Input: part model. Units: mm. Frame: model coordinates. Give positions to 0.01 mm unless a question says otherwise; leave off trailing zeros. Order: outer loops, then holes, each group sorted by start corner. A loop starts at its lowest first (then second) coordinate and runs counter-clockwise, first axis right, second up. Notation, with made-up numbers: M 4.5,-36 L 55.5,-36 A10 ccw 55.5,-25 Z; hole C 17.5,48 d1. An arc over 180 degrees is marked long. Use a Markdown table: item, result.
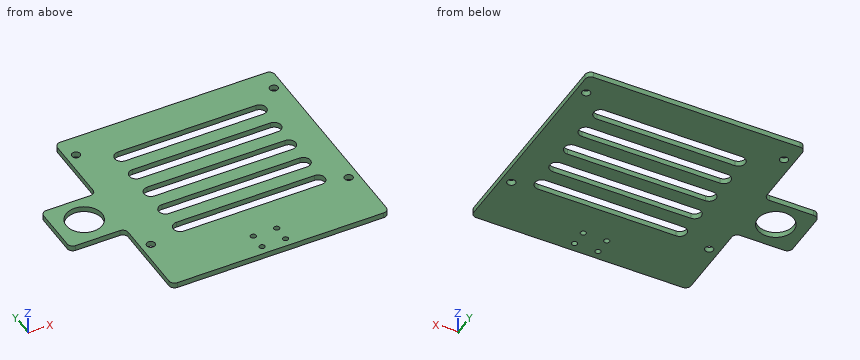
Autodesk Fusion 360 part; units mm, degrees
sketch "Sketch1" plane through (0, 0, 0) normal (0, 0, 1) x (1, 0, 0)
  line L0 (-78.5381, -2.5381) -> (-78.5381, 7.765)
  line L1 (-76.5381, 58.0111) -> (-1.7619, 58.0111)
  line L2 (0.2381, 56.0111) -> (0.2381, -2.5381)
  circle A0 centre (-3.3, -1) radius 1.5
  circle A1 centre (-3.3, 50) radius 1.5
  circle A2 centre (-75, 50) radius 1.5
  circle A3 centre (-75, -1) radius 1.5
  line L3 (-62.5, 45) -> (-12.5, 45)
  line L4 (-12.5, 40) -> (-62.5, 40)
  line L5 (-62.5, 35) -> (-12.5, 35)
  line L6 (-12.5, 30) -> (-62.5, 30)
  line L7 (-62.5, 25) -> (-12.5, 25)
  line L8 (-12.5, 20) -> (-62.5, 20)
  line L9 (-62.5, 15) -> (-12.5, 15)
  line L10 (-12.5, 10) -> (-62.5, 10)
  line L11 (-62.5, 5) -> (-12.5, 5)
  line L12 (-12.5, 0) -> (-62.5, 0)
  arc A4 (-62.5, 45) -> (-65, 42.5) centre (-62.5, 42.5) ccw
  arc A5 (-65, 42.5) -> (-62.5, 40) centre (-62.5, 42.5) ccw
  arc A6 (-10, 42.5) -> (-12.5, 45) centre (-12.5, 42.5) ccw
  arc A7 (-12.5, 40) -> (-10, 42.5) centre (-12.5, 42.5) ccw
  arc A8 (-62.5, 35) -> (-65, 32.5) centre (-62.5, 32.5) ccw
  arc A9 (-65, 32.5) -> (-62.5, 30) centre (-62.5, 32.5) ccw
  arc A10 (-10, 32.5) -> (-12.5, 35) centre (-12.5, 32.5) ccw
  arc A11 (-12.5, 30) -> (-10, 32.5) centre (-12.5, 32.5) ccw
  arc A12 (-10, 22.5) -> (-12.5, 25) centre (-12.5, 22.5) ccw
  arc A13 (-12.5, 20) -> (-10, 22.5) centre (-12.5, 22.5) ccw
  arc A14 (-62.5, 25) -> (-65, 22.5) centre (-62.5, 22.5) ccw
  arc A15 (-65, 22.5) -> (-62.5, 20) centre (-62.5, 22.5) ccw
  arc A16 (-62.5, 15) -> (-65, 12.5) centre (-62.5, 12.5) ccw
  arc A17 (-65, 12.5) -> (-62.5, 10) centre (-62.5, 12.5) ccw
  arc A18 (-10, 12.5) -> (-12.5, 15) centre (-12.5, 12.5) ccw
  arc A19 (-12.5, 10) -> (-10, 12.5) centre (-12.5, 12.5) ccw
  arc A20 (-10, 2.5) -> (-12.5, 5) centre (-12.5, 2.5) ccw
  arc A21 (-12.5, 0) -> (-10, 2.5) centre (-12.5, 2.5) ccw
  arc A22 (-62.5, 5) -> (-65, 2.5) centre (-62.5, 2.5) ccw
  arc A23 (-65, 2.5) -> (-62.5, 0) centre (-62.5, 2.5) ccw
  line L13 (-80.5381, 29.765) -> (-96.5381, 29.765)
  line L14 (-98.5381, 27.765) -> (-98.5381, 11.765)
  line L15 (-96.5381, 9.765) -> (-80.5381, 9.765)
  circle A24 centre (-88, 20) radius 6.5
  arc A25 (-76.5381, 58.0111) -> (-78.5381, 56.0111) centre (-76.5381, 56.0111) ccw
  arc A26 (0.2381, 56.0111) -> (-1.7619, 58.0111) centre (-1.7619, 56.0111) ccw
  arc A27 (-78.5381, 7.765) -> (-80.5381, 9.765) centre (-80.5381, 7.765) ccw
  arc A28 (-96.5381, 29.765) -> (-98.5381, 27.765) centre (-96.5381, 27.765) ccw
  arc A29 (-98.5381, 11.765) -> (-96.5381, 9.765) centre (-96.5381, 11.765) ccw
  line L16 (-78.5381, 56.0111) -> (-78.5381, 31.765)
  arc A30 (-80.5381, 29.765) -> (-78.5381, 31.765) centre (-80.5381, 31.765) ccw
  line L17 (0.2381, -2.5381) -> (0.2381, -19.9889)
  line L18 (-1.7619, -21.9889) -> (-76.5381, -21.9889)
  line L19 (-78.5381, -19.9889) -> (-78.5381, -2.5381)
  arc A31 (-78.5381, -19.9889) -> (-76.5381, -21.9889) centre (-76.5381, -19.9889) ccw
  arc A32 (-1.7619, -21.9889) -> (0.2381, -19.9889) centre (-1.7619, -19.9889) ccw
  circle A33 centre (-44.1028, -12.7273) radius 1
  circle A34 centre (-35.6028, -12.7273) radius 1
  circle A35 centre (-35.6028, -18.7273) radius 1
  circle A36 centre (-44.1028, -18.7273) radius 1
  point P0 (-98.5381, 29.765)
  dimension "d1" = 71.7
  dimension "d2" = 51
  dimension "d4" = 3
  dimension "d5" = 3
  dimension "d6" = 3
  dimension "d7" = 3
  dimension "d8" = 2.5
  dimension "d9" = 2.5
  dimension "d18" = 13
  dimension "d21" = 2
  dimension "d22" = 2
  dimension "d25" = 2
  dimension "d28" = 80
  dimension "d37" = 8.5
  dimension "d38" = 6
  dimension "d39" = 2
  dimension "d40" = 2
  dimension "d41" = 2
  dimension "d42" = 2
extrude "Extrude4" add sketch "Sketch1" along normal blind 2
1) Cut plane D-D on z = 1.65. State how many separate pieces and enclosed holes the cut face has, and give its area (3 significant figures).
Response values:
| item | result |
|---|---|
| separate pieces | 1 |
| enclosed holes | 14 |
| area | 5,180 mm² |
2) Cut plane C-C on y = 22.5. Return loops of the section in (x, z), and give its area (3 significant figures).
Response values:
| item | result |
|---|---|
| outline | M -98.54,0 L -94,0 L -94,2 L -98.54,2 Z; M -82,0 L -65,0 L -65,2 L -82,2 Z; M -10,0 L 0.24,0 L 0.24,2 L -10,2 Z |
| area | 63.6 mm² |
3) Cut plane A-A on y = 50. Return loops of the section in (x, z), and give its area (3 significant figures).
Response values:
| item | result |
|---|---|
| outline | M -78.54,0 L -76.5,0 L -76.5,2 L -78.54,2 Z; M -73.5,0 L -4.8,0 L -4.8,2 L -73.5,2 Z; M -1.8,0 L 0.24,0 L 0.24,2 L -1.8,2 Z |
| area | 146 mm² |
4) Material intervals for line 1 (Y direction, x = -56, z = 1.15); line 2 (Y direction, x = -88.5, z = 0.35) (3 decimals); line 3 (X direction, y = 21, z = 1), sorted ascending. Write a range as from..to.
Response values:
| item | result |
|---|---|
| line 1 | y = -21.99..0, 5..10, 15..20, 25..30, 35..40, 45..58.01 |
| line 2 | y = 9.765..13.519, 26.481..29.765 |
| line 3 | x = -98.54..-94.42, -81.58..-64.5, -10.5..0.24 |
5) Cut plane B-B on y = 2.5. Return loops of the section in (x, z).
Response values:
| item | result |
|---|---|
| outline | M -78.54,0 L -65,0 L -65,2 L -78.54,2 Z; M -10,0 L 0.24,0 L 0.24,2 L -10,2 Z |
6) First-contact query: pin 1 Ø2.5 at (x, y) = (-75, -1) entering from -Z; pin 2 Ø0.6 at (y, z) = (0.5, 1) entering from -X. Flat tips, straight axial feed; report the tip coordinate or a pass-through.
Response values:
| item | result |
|---|---|
| pin 1 | passes through |
| pin 2 | stops at x = -78.54 |
